The model under review builds one solid part; all positions refer to its coordinate system, in mm. Round coordinates to 2 decimals unless told otherwise and drop trailing zeros. Order: outer loops, then holes, each group sorted by start corner. A loop starts at its lowest first (then second) coordinate and runs counter-clockwise, first axis right, second up.
1) Mouldability with a two-part tool opening along Z and no side actions: class faces 1 (the face through (651.15, 26.13, 8.23)), 2 (the face through (651.15, 28.77, 9.06)), 3 (the face through (0, 7, -27)) as pulls with the +Z half, pulls with the -Z half, needs draft (parallel to the pull), parting line crosses it, or undercut.
2) Consider section C-C (x = 809). Give the boundary of the cut face in (y, z) (1 decimal), then the cut area to 3 significant figures.
3) Consider section B-B (x = 245). Give the boundary of the cut face in (y, z) (1 decimal).
4) Clearance check with flat-ended pins moving along their axes: P1, Ø6.5, axis at x = 85.725, z = 0, coming from the +Y side; P2, Ø6, axis at x = 665, y = -7, coming from the +Z side; P3, Ø5, axis at x = 1163.5, y = 3.5, coming from the -Z side; P4, Ø4.5, axis at x = 473.075, z = 0, coming from the +Y side. State where each tip first meets the part, or that it passes through.
5) Consider section A-A (y = 0). Give the boundary of the cut face in (x, z), then the cut area to 3 significant figures.
6) To check wall thickness, follow L1, parallel to X at y = -25, z = 16.5 (3 decimals); L2, parallel to Z at x = 597, y = 0; L3, parallel to Z at x = 875, y = 3.5. State the ranges of each line that lie inside material, in increasing order.
from build123d import *

# Parameters (mm, degrees)
F0_R     = 30.1625
F0_R_2   = 27.3939
F1_DEPTH = 1320.8
F4_DEPTH = 450.85
F5_R     = 3.175
F6_DEPTH = 76.2
F7_R     = 2.5527
F8_DEPTH = 76.2


with BuildPart() as f1:
    # F0 (on Right) → F1 (new body)
    with BuildSketch(Plane.YZ):
        Circle(F0_R)
        Circle(F0_R_2, mode=Mode.SUBTRACT)
    extrude(amount=F1_DEPTH)

    # F3 (on offset) → F4 (cut)
    with BuildSketch(Plane(origin=(53.975, 0, 0), x_dir=(0, -1, 0), z_dir=(-1, 0, 0))):
        Polygon((28.7277697928, 42.2795656081), (0, 0), (35.903159529, 0), align=None)
        Polygon((35.903159529, 0), (0, 0), (28.4545668533, -41.8774842184), align=None)
    extrude(amount=-F4_DEPTH, mode=Mode.SUBTRACT)

    # F5 (on Front) → F6 (cut)
    with BuildSketch(Plane.XZ):
        with Locations((47.625, 0)):
            Circle(F5_R)
        with Locations((511.175, 0)):
            Circle(F5_R)
    extrude(amount=F6_DEPTH, mode=Mode.SUBTRACT)

    # F7 (on Front) → F8 (cut)
    with BuildSketch(Plane.XZ):
        with Locations((85.725, 0)):
            Circle(F7_R)
        with Locations((473.075, 0)):
            Circle(F7_R)
    extrude(amount=-F8_DEPTH, mode=Mode.SUBTRACT)


solid = f1.part
Answer below:
1. face 1: undercut
1. face 2: parting line crosses it
1. face 3: needs draft
2. outline: circle Ø60.3 at (0, 0); hole circle Ø54.8 at (0, 0)
2. area: 501 mm2
3. outline: (-17, -24.9) arc R30.2 ccw (long way) to (-17, 24.9) - (-15.4, 22.7) arc R27.4 cw (long way) to (-15.4, -22.7) - close
4. P1: stops at y = 30.16
4. P2: stops at z = 29.9
4. P3: stops at z = -30.15
4. P4: passes through
5. outline: (0, -30.16) - (1320.8, -30.16) - (1320.8, -27.39) - (0, -27.39) - close; (0, 27.39) - (1320.8, 27.39) - (1320.8, 30.16) - (0, 30.16) - close
5. area: 7,310 mm2
6. L1: x = 0 to 53.975, 504.825 to 1320.8
6. L2: z = -30.16 to -27.39, 27.39 to 30.16
6. L3: z = -29.96 to -27.17, 27.17 to 29.96
